Study the drawing (mm; zero at the part's minimum x, y, z) and answer. A direction names the side the tool comes from. Coordinates: 2 decimals unless noted, no trailing zeros. Loops run counter-clockwise (first coordinate to the right, second up) from the corner with the lowest first, then second, coordinate; pieces in that order, holes last. Notation, with made-up numbers: (35, 39) - (63, 39) arc R31 ccw to (63, 77) - close; hole circle Ø8 at (42.5, 3). An arc over 180 degrees is marked (long way). Use one line per item in the form item = value. Start each with the question number.
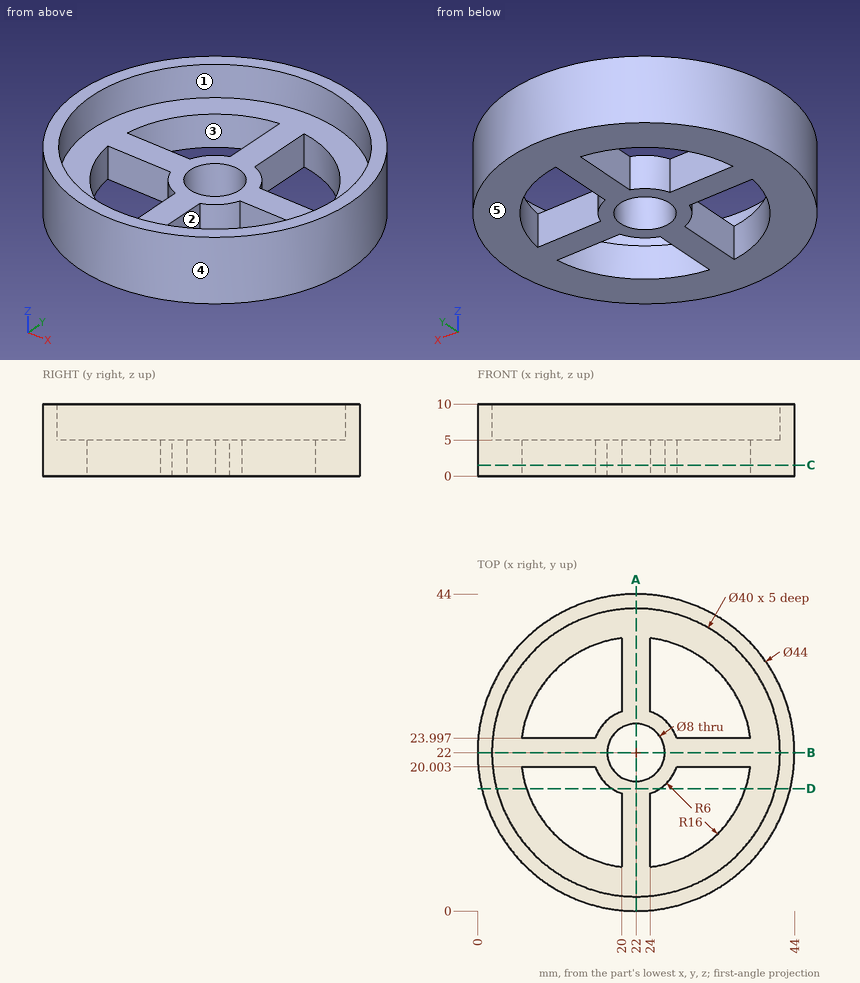
(1) A cutting plane is placed at C-C (z = 1.5). Determine the outline of the cut face in (x, y) (1 decimal), then the cut area to 3 significant figures.
(2) A cutting plane is placed at D-D (y = 17). Determine the outline of the cut face in (x, z) (1 decimal).
(3) Find the intervals of material crossed by probe 1 along Y at (x, z) = (22, 8.05); probe 2 along Y at (x, z) = (22, 1.65); probe 3 along X at (y, z) = (31.5, 4.25) (1 decimal), in increasing order. Write a range as from..to.
(4) Determine the mould class of the marked faces 3, 4 and 5 for opening direction Y: +Y half, -Y half, draft (parallel to the pull), parting line (faces both ways), or undercut.
(5) Each of these flat-tipped pins is pushed along its axis until it touches: pin 1 Ø4 at (y, z) = (10, 1.5) entering from +X; pin 2 Ø1.5 at (x, z) = (11, 3.5) entering from +Y; pin 3 Ø5.5 at (y, z) = (31, 1.5) entering from -X. Where does it stop, or does it pass through?
(6) For the marked faces 1 and 2, determine the directions among +Z, -Z, +X, -X, +Y, -Y from which every point of the face is accessible in a straight line to the end or side of a thin tool.
(7) A cutting plane is placed at A-A (x = 22). Determine the outline of the cut face in (y, z).
Evaluation:
q1.outline = circle Ø44 at (22, 22); hole (6.1, 20) arc R16 ccw to (20, 6.1) - (20, 16.3) arc R6 cw to (16.3, 20) - close; hole (6.1, 24) - (16.3, 24) arc R6 cw to (20, 27.7) - (20, 37.9) arc R16 ccw to start; hole circle Ø8 at (22, 22); hole (24, 6.1) arc R16 ccw to (37.9, 20) - (27.7, 20) arc R6 cw to (24, 16.3) - close; hole (24, 27.7) arc R6 cw to (27.7, 24) - (37.9, 24) arc R16 ccw to (24, 37.9) - close
q1.area = 940 mm^2
q2.outline = (0.6, 0) - (6.8, 0) - (6.8, 5) - (2.6, 5) - (2.6, 10) - (0.6, 10) - close; (18.7, 0) - (25.3, 0) - (25.3, 5) - (18.7, 5) - close; (37.2, 0) - (43.4, 0) - (43.4, 10) - (41.4, 10) - (41.4, 5) - (37.2, 5) - close
q3.probe_1 = 0..2, 42..44
q3.probe_2 = 0..18, 26..44
q3.probe_3 = 2.2..9.1, 20..24, 34.9..41.8
q4.face_3 = undercut
q4.face_4 = parting line
q4.face_5 = draft
q5.pin_1 = 41.6
q5.pin_2 = 41.47
q5.pin_3 = 0.91
q6.face_1 = +Z
q6.face_2 = +Z, -Z
q7.outline = (0, 0) - (18, 0) - (18, 5) - (2, 5) - (2, 10) - (0, 10) - close; (26, 0) - (44, 0) - (44, 10) - (42, 10) - (42, 5) - (26, 5) - close
